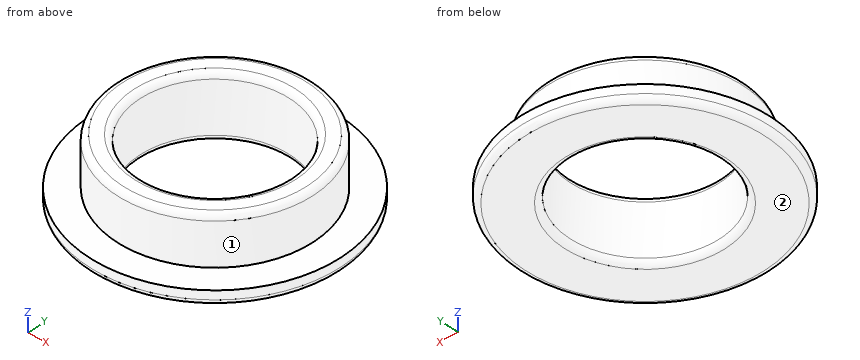
```python
from build123d import *

# Parameters (mm, degrees)
F0_R     = 33.02
F0_R_2   = 19.685
F1_DEPTH = 3.81
F2_R     = 25.781
F2_R_2   = 19.685
F3_DEPTH = 12.7
F4_R     = 1.524


with BuildPart() as f1:
    # F0 (on Top) → F1 (new body)
    with BuildSketch(Plane.XY):
        Circle(F0_R)
        Circle(F0_R_2, mode=Mode.SUBTRACT)
    extrude(amount=F1_DEPTH)

    # F2 (on face) → F3 (join)
    with BuildSketch(Plane.XY.offset(3.81)):
        Circle(F2_R)
        Circle(F2_R_2, mode=Mode.SUBTRACT)
    extrude(amount=F3_DEPTH)

    # F4
    f4_edges = [f1.edges().sort_by_distance(p)[0] for p in [
        (-33.02, 0, 0),
        (-19.685, 0, 0),
        (-25.781, 0, 16.51),
        (-19.685, 0, 16.51),
    ]]
    fillet(f4_edges, radius=F4_R)


solid = f1.part
```
Work out the finished part from the listing and answer in its coordinate system (mm). Face numbers are marked on the shaded views. A direction names the side the tool comes from. Coordinates: 2 decimals unless noted, no trailing zeros. Loops run counter-clockwise (first coordinate to the right, second up) from the corner with the lowest first, then second, coordinate; pieces in that order, holes last.
1) Flat-ended cylindrical pins translate along their axes: pin 1 (5 mm diameter, centred on x = -2, z = 6, fed in from -Y); pin 2 (5 mm diameter, centred on x = 0, z = 8, fed in from -Y). Find the tip coordinate at first contact, or state that the pin passes through.
Results:
pin 1: stops at y = -33.01
pin 2: stops at y = -25.78
2) Consider probe 1 along Y at (x, z) = (0, 10) (3 decimals); probe 2 along X at (y, z) = (-0.5, 6); probe 3 along Z at (x, y) = (19.5, -24). Determine where each line is inside the solid, lowest interval first.
Results:
probe 1: y = -25.781 to -19.685, 19.685 to 25.781
probe 2: x = -25.78 to -19.68, 19.68 to 25.78
probe 3: z = 0 to 3.81
3) For the marked faces 1 and 2, determine the directions among +Z, -Z, +X, -X, +Y, -Y from which every point of the face is accessible in a straight line to the end or side of a thin tool.
Results:
face 1: +Z
face 2: -Z, +X, -X, +Y, -Y
4) Section C-C (z = 10) is taken. Give the vertices of the cut face in (x, y) (3 decimals), plus the area to 3 significant figures.
Results:
outline: circle Ø51.562 at (0, 0); hole circle Ø39.37 at (0, 0)
area: 871 mm2
5) Section A-A (y = 0) is taken. Give the vertices of the cut face in (x, z) (3 decimals).
Results:
outline: (-33.02, 1.524) arc R1.524 ccw to (-31.496, 0) - (-21.209, 0) arc R1.524 ccw to (-19.685, 1.524) - (-19.685, 14.986) arc R1.524 ccw to (-21.209, 16.51) - (-24.257, 16.51) arc R1.524 ccw to (-25.781, 14.986) - (-25.781, 3.81) - (-33.02, 3.81) - close; (19.685, 1.524) arc R1.524 ccw to (21.209, 0) - (31.496, 0) arc R1.524 ccw to (33.02, 1.524) - (33.02, 3.81) - (25.781, 3.81) - (25.781, 14.986) arc R1.524 ccw to (24.257, 16.51) - (21.209, 16.51) arc R1.524 ccw to (19.685, 14.986) - close
